Part model, mm, in its own coordinate system. Face numbers are marked on the shaded views. Round coordinates to 2 decimals unless told otherwise and drop trailing zeros. Order: outer loops, then holes, each group sorted by start corner. A loop starts at its lowest first (then second) coordinate and runs counter-clockwise, first axis right, second up. Notation, with made-up numbers: (48, -12) -> (97, -12) arc R19 ccw to (97, 10) -> close; hole circle Ø9 at (17.5, 50). An arc over 180 degrees is marked (long way). Return JSON: item names as keys, results as strings. Group by question number.
from build123d import *

# Parameters (mm, degrees)
ESQUISSE1_R             = 5
BOSS_EXTRU_1_DEPTH      = 0.5
ESQUISSE2_R             = 4.5
ESQUISSE2_R_2           = 4
ESQUISSE2_R_3           = 3.5
ESQUISSE2_R_4           = 3
ESQUISSE2_R_5           = 2.5
ESQUISSE2_R_6           = 2
ESQUISSE2_R_7           = 1.5
ESQUISSE2_R_8           = 1
ESQUISSE2_R_9           = 0.5
ENL_V_MAT_EXTRU_2_DEPTH = 0.2
CHANFREIN1_SIZE         = 0.5
CHANFREIN1_SIZE_2       = 0.202013113


with BuildPart() as part:
    # Esquisse1 → Boss.-Extru.1 (new body)
    with BuildSketch(Plane.XY):
        Circle(ESQUISSE1_R)
    extrude(amount=BOSS_EXTRU_1_DEPTH)

    # Esquisse2 → Enlèv. mat.-Extru.2 (cut)
    # profile 1 of 5: a face of its own
    with BuildSketch(Plane.XY.offset(0.5)):
        Circle(ESQUISSE2_R)
        Circle(ESQUISSE2_R_2, mode=Mode.SUBTRACT)
    # profile 2 of 5: a face of its own
    with BuildSketch(Plane.XY.offset(0.5)):
        Circle(ESQUISSE2_R_3)
        Circle(ESQUISSE2_R_4, mode=Mode.SUBTRACT)
    # profile 3 of 5: a face of its own
    with BuildSketch(Plane.XY.offset(0.5)):
        Circle(ESQUISSE2_R_5)
        Circle(ESQUISSE2_R_6, mode=Mode.SUBTRACT)
    # profile 4 of 5: a face of its own
    with BuildSketch(Plane.XY.offset(0.5)):
        Circle(ESQUISSE2_R_7)
        Circle(ESQUISSE2_R_8, mode=Mode.SUBTRACT)
    # profile 5 of 5: a face of its own
    with BuildSketch(Plane.XY.offset(0.5)):
        Circle(ESQUISSE2_R_9)
    extrude(amount=-ENL_V_MAT_EXTRU_2_DEPTH, mode=Mode.SUBTRACT)

    # Chanfrein1
    # the kernel refuses this chamfer: 0.5, 0.202013113 mm, written as the material it takes off along each edge
    with BuildSketch(Plane(origin=(0, 0, 0.5), x_dir=(1, 0, 0), z_dir=(0, -1, 0))) as chanfrein1_piece_1_section:
        Polygon((0.5 + CHANFREIN1_SIZE, 0), (0.5, -CHANFREIN1_SIZE_2), (0.5, 0), align=None)
    chanfrein1_piece_1 = revolve(axis=Axis((0, 0, 0.5), (0, 0, 1)), mode=Mode.PRIVATE)
    chanfrein1_piece_1 = split(chanfrein1_piece_1, bisect_by=Plane(origin=(-0.759410198, 0, 0.3), z_dir=(0, 0, 1)), keep=Keep.TOP, mode=Mode.PRIVATE)
    add(chanfrein1_piece_1, mode=Mode.SUBTRACT)
    with BuildSketch(Plane(origin=(0, 0, 0.5), x_dir=(1, 0, 0), z_dir=(0, -1, 0))) as chanfrein1_piece_2_section:
        Polygon((1.5 + CHANFREIN1_SIZE, 0), (1.5, -CHANFREIN1_SIZE_2), (1.5, 0), align=None)
    chanfrein1_piece_2 = revolve(axis=Axis((0, 0, 0.5), (0, 0, 1)), mode=Mode.PRIVATE)
    chanfrein1_piece_2 = split(chanfrein1_piece_2, bisect_by=Plane(origin=(-1.758573668, 0, 0.3), z_dir=(0, 0, 1)), keep=Keep.TOP, mode=Mode.PRIVATE)
    add(chanfrein1_piece_2, mode=Mode.SUBTRACT)
    with BuildSketch(Plane(origin=(0, 0, 0.5), x_dir=(1, 0, 0), z_dir=(0, -1, 0))) as chanfrein1_piece_3_section:
        Polygon((2.5 + CHANFREIN1_SIZE, 0), (2.5, -CHANFREIN1_SIZE_2), (2.5, 0), align=None)
    chanfrein1_piece_3 = revolve(axis=Axis((0, 0, 0.5), (0, 0, 1)), mode=Mode.PRIVATE)
    chanfrein1_piece_3 = split(chanfrein1_piece_3, bisect_by=Plane(origin=(-2.75803387, 0, 0.3), z_dir=(0, 0, 1)), keep=Keep.TOP, mode=Mode.PRIVATE)
    add(chanfrein1_piece_3, mode=Mode.SUBTRACT)
    with BuildSketch(Plane(origin=(0, 0, 0.5), x_dir=(1, 0, 0), z_dir=(0, -1, 0))) as chanfrein1_piece_4_section:
        Polygon((3.5 + CHANFREIN1_SIZE, 0), (3.5, -CHANFREIN1_SIZE_2), (3.5, 0), align=None)
    chanfrein1_piece_4 = revolve(axis=Axis((0, 0, 0.5), (0, 0, 1)), mode=Mode.PRIVATE)
    chanfrein1_piece_4 = split(chanfrein1_piece_4, bisect_by=Plane(origin=(-3.757616815, 0, 0.3), z_dir=(0, 0, 1)), keep=Keep.TOP, mode=Mode.PRIVATE)
    add(chanfrein1_piece_4, mode=Mode.SUBTRACT)
    with BuildSketch(Plane(origin=(0, 0, 0.5), x_dir=(1, 0, 0), z_dir=(0, -1, 0))) as chanfrein1_piece_5_section:
        Polygon((4.5 + CHANFREIN1_SIZE, 0), (4.5, -CHANFREIN1_SIZE_2), (4.5, 0), align=None)
    chanfrein1_piece_5 = revolve(axis=Axis((0, 0, 0.5), (0, 0, 1)), mode=Mode.PRIVATE)
    chanfrein1_piece_5 = split(chanfrein1_piece_5, bisect_by=Plane(origin=(-4.757270103, 0, 0.3), z_dir=(0, 0, 1)), keep=Keep.TOP, mode=Mode.PRIVATE)
    add(chanfrein1_piece_5, mode=Mode.SUBTRACT)


solid = part.part
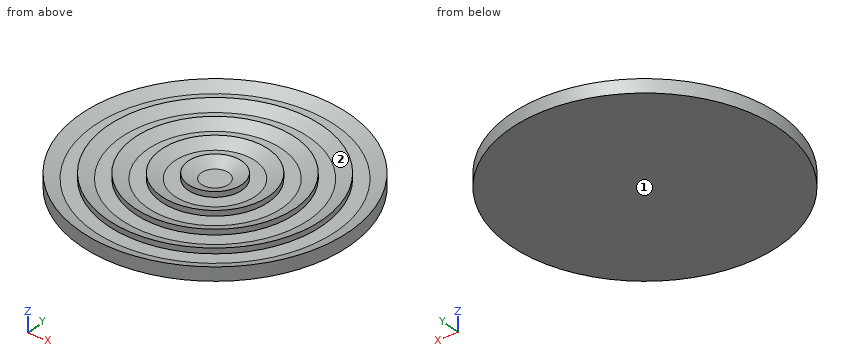
(1) Probe L1, parallel to Z at x = 1.75, y = -1.25; L2, parallel to X at y = -2, z = 0.15; L3, parallel to Y at x = 3.75, z = 0.25. List the from-to ranges inside material, lowest first. Write a range as [from, to].
(2) Mould opens along X. For the marked faces 1 and 2 say: pulls with the +X half, pulls with the -X half, needs draft (parallel to the pull), parting line crosses it, or undercut.
(3) Pin check, flat tips, straight feed: P1, Ø3, axis at x = -4, y = 2, coming from the +Z side; P2, Ø0.8, axis at x = 0, y = 0, coming from the +Z side. Stop position of each tip, or through.
(4) Saw through at C-C, the plane z = 0.2. List the corners of the cut face in (x, y), and give its area (3 significant figures).
Results are:
{
 "1": {"L1": "z = [0, 0.3]", "L2": "x = [-4.58, 4.58]", "L3": "y = [-3.31, 3.31]"},
 "2": {"face 1": "needs draft", "face 2": "undercut"},
 "3": {"P1": "stops at z = 0.5", "P2": "stops at z = 0.3"},
 "4": {"outline": "circle Ø10 at (0, 0)", "area": "78.5 mm^2"}
}
